For this review, take the finished solid that the model builds, in its own axes (mm). A direction names the side the tool comes from. Round coordinates to 2 decimals unless told otherwise and drop trailing zeros. Order: outer loops, then holes, each group sorted by start corner. A loop starts at its lowest first (then second) coordinate and runs counter-clockwise, first axis right, second up. Notation, with made-up numbers: (62, 85) -> (86, 85) arc R26 ccw to (86, 119) -> close; hole circle Ø2 at (67, 27). An arc over 180 degrees is marked (long way). Answer in a Markdown table with one row per item.
```python
from build123d import *

# Parameters (mm, degrees)
SKETCH_1_R             = 17.5
EXTRUDE_1_DEPTH        = 47.6
SKETCH_2_R             = 9.5
CUT_EXTRUDE_1_DEPTH    = 1
SKETCH_3_R             = 10.5
SKETCH_3_R_2           = 9.5
EXTRUDE_2_DEPTH        = 1.7
SKETCH_4_R             = 5
EXTRUDE_3_DEPTH        = 26
CUT_EXTRUDE_2_DEPTH    = 20
SKETCH_12_R            = 15
EXTRUDE_4_DEPTH        = 67
EXTRUDE_5_DEPTH        = 19
HOLE_WIZARD_M4_6_D     = 3.3
HOLE_WIZARD_M4_6_DEPTH = 8
HOLE_WIZARD_M4_6_TIP   = 0.991420021
SKETCH_18_R            = 17.5
SKETCH_18_R_2          = 17
CUT_EXTRUDE_5_DEPTH    = 0.5
SKETCH_19_R            = 17.5
SKETCH_19_R_2          = 17
CUT_EXTRUDE_6_DEPTH    = 0.5
SKETCH_20_R            = 15
SKETCH_20_R_2          = 14.75
CUT_EXTRUDE_7_DEPTH    = 0.5
CHAMFER_1_SIZE         = 0.3
CHAMFER_2_SIZE         = 0.3
FILLET_1_R             = 5


with BuildPart() as part:
    # 草图1 → 凸台-拉伸1 (new body)
    with BuildSketch(Plane.XY):
        Circle(SKETCH_1_R)
    extrude(amount=EXTRUDE_1_DEPTH)

    # 草图2 → 切除-拉伸1 (cut)
    with BuildSketch(Plane.XY.offset(47.6)):
        Circle(SKETCH_2_R)
    extrude(amount=-CUT_EXTRUDE_1_DEPTH, mode=Mode.SUBTRACT)

    # 草图3 → 凸台-拉伸2 (add)
    with BuildSketch(Plane.XY.offset(47.6)):
        Circle(SKETCH_3_R)
        Circle(SKETCH_3_R_2, mode=Mode.SUBTRACT)
    extrude(amount=EXTRUDE_2_DEPTH)

    # 草图4 → 凸台-拉伸3 (add)
    with BuildSketch(Plane.XY.offset(46.6)):
        Circle(SKETCH_4_R)
    extrude(amount=EXTRUDE_3_DEPTH)

    # 草图5 → 切除-拉伸2 (cut)
    with BuildSketch(Plane.XY.offset(72.6)):
        with BuildLine():
            Line((-3.469870315, -3.6), (3.469870315, -3.6))
            ThreePointArc((3.469870315, -3.6), (0, -5), (-3.469870315, -3.6))
        make_face()
    extrude(amount=-CUT_EXTRUDE_2_DEPTH, mode=Mode.SUBTRACT)

    # 草图12 → 凸台-拉伸4 (add)
    with BuildSketch(Plane(origin=(0, 0, 0), x_dir=(-1, 0, 0), z_dir=(0, 0, -1))):
        Circle(SKETCH_12_R)
    extrude(amount=EXTRUDE_4_DEPTH)

    # 草图15 → 凸台-拉伸5 (add)
    with BuildSketch(Plane(origin=(0, 0, -67), x_dir=(-1, 0, 0), z_dir=(0, 0, -1))):
        with BuildLine():
            Line((-15, 0), (-15, -25))
            Line((-15, -25), (15, -25))
            Line((15, -25), (15, 0))
            ThreePointArc((15, 0), (0, 15), (-15, 0))
        make_face()
    extrude(amount=EXTRUDE_5_DEPTH)

    # M4 螺纹孔6
    with Locations(Plane(origin=(0, 14, 47.6), x_dir=(1, 0, 0), z_dir=(0, 0, 1))):
        with Locations((0, 0), (-9.899494937, -4.100505063), (-14, -14), (-9.899494937, -23.899494937), (0, -28), (9.899494937, -23.899494937), (14, -14), (9.899494937, -4.100505063)):
            Hole(HOLE_WIZARD_M4_6_D / 2, depth=HOLE_WIZARD_M4_6_DEPTH)
            with Locations((0, 0, -(HOLE_WIZARD_M4_6_DEPTH + HOLE_WIZARD_M4_6_TIP / 2))):  # 118° drill point
                Cone(0, HOLE_WIZARD_M4_6_D / 2, HOLE_WIZARD_M4_6_TIP, mode=Mode.SUBTRACT)

    # 草图18 → 切除-拉伸5 (cut)
    with BuildSketch(Plane.XY.offset(41.6)):
        Circle(SKETCH_18_R)
        Circle(SKETCH_18_R_2, mode=Mode.SUBTRACT)
    extrude(amount=-CUT_EXTRUDE_5_DEPTH, mode=Mode.SUBTRACT)

    # 草图19 → 切除-拉伸6 (cut)
    with BuildSketch(Plane(origin=(0, 0, 8), x_dir=(-1, 0, 0), z_dir=(0, 0, -1))):
        Circle(SKETCH_19_R)
        Circle(SKETCH_19_R_2, mode=Mode.SUBTRACT)
    extrude(amount=-CUT_EXTRUDE_6_DEPTH, mode=Mode.SUBTRACT)

    # 草图20 → 切除-拉伸7 (cut)
    with BuildSketch(Plane.XY.offset(-67)):
        Circle(SKETCH_20_R)
        Circle(SKETCH_20_R_2, mode=Mode.SUBTRACT)
    extrude(amount=CUT_EXTRUDE_7_DEPTH, mode=Mode.SUBTRACT)

    # 倒角1
    chamfer_1_edges = [part.edges().sort_by_distance(p)[0] for p in [
        (-17.5, 0, 0),
        (-1.955843607, 4.601594918, 72.6),
        (-17.5, 0, 47.6),
    ]]
    chamfer(chamfer_1_edges, length=CHAMFER_1_SIZE)

    # 倒角2
    chamfer_2_edges = [part.edges().sort_by_distance(p)[0] for p in [
        (-10.5, 0, 49.3),
    ]]
    chamfer(chamfer_2_edges, length=CHAMFER_2_SIZE)

    # 圆角1
    fillet_1_edges = [part.edges().sort_by_distance(p)[0] for p in [
        (15, -25, -76.5),
        (-15, -25, -76.5),
    ]]
    fillet(fillet_1_edges, radius=FILLET_1_R)


solid = part.part
```
Q1. Tool access review of faces 1 (the face through (-9.139, 14.334, 8.246)), 2 (the face through (15, -10, -76)), 3 (the face through (10.3, 8.3, 43.5)), 4 (the face through (0, 1, 72.6)): name each direction out of +Z, -Z, +X, -X, +Y, -Y from which nothing blocks a thin tool from reaching the whole face with its end or side.
Answer key:
| item | result |
|---|---|
| face 1 | none |
| face 2 | -Z, +X, +Y, -Y |
| face 3 | +Z |
| face 4 | +Z, +X, -X, +Y, -Y |
Q2. The part is to be moulded in two halves that separate along Y. For faces 5 (the face through (7, -7, 49.3)), 6 (the face through (13.714, 0.013, 38.781)), 7 (the face through (0, 15, -76)), 8 (the face through (-9.94, 10.18, 38.78)), say which applies: +Y half, -Y half, draft (parallel to the pull), parting line (faces both ways), or undercut.
Answer key:
| item | result |
|---|---|
| face 5 | draft |
| face 6 | undercut |
| face 7 | +Y half |
| face 8 | undercut |
Q3. To check wall thickness, follow probe 1 along Y at (x, z) = (0, 45); probe 2 along X at (y, z) = (1.5, 45.5); probe 3 along Z at (x, y) = (-13.5, -21.5). State the ranges of each line that lie inside material, in increasing order.
Answer key:
| item | result |
|---|---|
| probe 1 | y = -17.5 to -15.65, -12.35 to 12.35, 15.65 to 17.5 |
| probe 2 | x = -17.44 to -14.69, -13.31 to 13.31, 14.69 to 17.44 |
| probe 3 | z = -86 to -67 |
Q4. Clearance check with flat-ended pins moving along their axes: pin 1 Ø1 at (y, z) = (-3.5, -13.5) entering from +X; pin 2 Ø21 at (y, z) = (-11.5, -74.5) entering from -X; pin 3 Ø1 at (x, z) = (6.5, -29) entering from -Y. State where each tip first meets the part, or that it passes through.
Answer key:
| item | result |
|---|---|
| pin 1 | stops at x = 14.7 |
| pin 2 | stops at x = -15 |
| pin 3 | stops at y = -13.75 |
Q5. Take a section at A-A, the plane z = -55.5. Write out the cut boundary in (x, y).
Answer key:
| item | result |
|---|---|
| outline | circle Ø30 at (0, 0) |
